from build123d import *

# Parameters (mm, degrees)
SKETCH_1_R          = 10
EXTRUDE_1_DEPTH     = 15
SKETCH_2_R          = 9
SKETCH_2_R_2        = 4
CUT_EXTRUDE_1_DEPTH = 1
FILLET_1_R          = 0.5
SKETCH_3_R          = 2
CUT_EXTRUDE_2_DEPTH = 8


with BuildPart() as part:
    # 草图1 → 凸台-拉伸1 (new body)
    with BuildSketch(Plane.XY):
        Circle(SKETCH_1_R)
    extrude(amount=EXTRUDE_1_DEPTH)

    # 草图2 → 切除-拉伸1 (cut)
    with BuildSketch(Plane.XY.offset(15)):
        Circle(SKETCH_2_R)
        Circle(SKETCH_2_R_2, mode=Mode.SUBTRACT)
    extrude(amount=-CUT_EXTRUDE_1_DEPTH, mode=Mode.SUBTRACT)

    # 圆角1
    fillet_1_edges = [part.edges().sort_by_distance(p)[0] for p in [
        (-10, 0, 0),
        (-10, 0, 15),
        (-9, 0, 15),
    ]]
    fillet(fillet_1_edges, radius=FILLET_1_R - 0.0001)  # a hair under: the kernel refuses the full size

    # 草图3 → 切除-拉伸2 (cut)
    with BuildSketch(Plane(origin=(0, 0, 0), x_dir=(-1, 0, 0), z_dir=(0, 0, -1))):
        Circle(SKETCH_3_R)
    extrude(amount=-CUT_EXTRUDE_2_DEPTH, mode=Mode.SUBTRACT)


solid = part.part
Geometry: final body of the model. Coordinates: model frame, mm. A direction names the side the tool comes from. Coordinates: 2 decimals unless noted, no trailing zeros. Loops run counter-clockwise (first coordinate to the right, second up) from the corner with the lowest first, then second, coordinate; pieces in that order, holes last. Notation, with made-up numbers: M 18,16 L 48,16 A5 ccw 48,25 Z; hole C 32,42.25 d2. An arc over 180 degrees is marked long. One line per item, written item: value. Start each with the question number.
1) Reachability of faces 1 (the cylindrical face through (-0.867, -3.905, 14.507)), 2 (the cylindrical face through (0, -2, 4)), 3 (the cylindrical face through (-2.17, -9.76, 7.4)) from +Z, -Z, +X, -X, +Y, -Y: full face, straight path, thin tool, end or side. Return the list, or none.
2) Cut plane C-C (z = 6.5). Return loops of the section in (x, y), then the cut area to 3 significant figures.
3) Material intervals for L1, parallel to Y at x = 0, z = 14.1; L2, parallel to Y at x = 0, z = 2.25; L3, parallel to Z at x = 3.75, y = -6.5, sorted ascending. Write a range as from..to.
4) Pin query (flat end, axial travel): P1, Ø3, axis at x = 0.5, y = 1, coming from the -Z side; P2, Ø3, axis at x = 2.5, z = 2.5, coming from the -Y side; P3, Ø5, axis at y = -8, z = 2, coming from the -X side; P4, Ø1, axis at y = -1, z = 5.5, coming from the -X side. Return the tip coordinate at first contact, or that it passes through.
5) Cut plane D-D (z = 10.75). Return loops of the section in (x, y).
Evaluation:
1. face 1: +Z
1. face 2: -Z
1. face 3: +Z, -Z
2. outline: C 0,0 d20; hole C 0,0 d4
2. area: 302 mm^2
3. L1: -10..-9, -4..4, 9..10
3. L2: -10..-2, 2..10
3. L3: 0..14
4. P1: z = 0
4. P2: y = -9.95
4. P3: x = -8.35
4. P4: x = -9.99
5. outline: C 0,0 d20
